Geometry check sheet. Reference: drawing and pictorial views, mm from the part's lowest x, y, z. A direction names the side the tool comes from. Round coordinates to 2 decimals unless told otherwise and drop trailing zeros. Write each loop counter-clockwise with the first axis right and the second up, starting at its lowest first coordinate (ties: lowest second). Pieces come first, ordered by that corner, then holes. Notation, with made-up numbers: M -6.75,17 L 9.25,17 A15 cw 9.25,41 Z; hole C 87.25,-5 d10. An arc over 180 degrees is marked long. Answer in a Markdown table with one row per item. Add a question column.
1. Go/stop test with flat-tipped pins: pin 1 Ø10 at (y, z) = (6, 25) entering from +X; pin 2 Ø6 at (x, z) = (5, 22) entering from -Y; pin 3 Ø12 at (y, z) = (24.5, 28) entering from -X. Record where each tip stops, or that it passes through.
2. Material ranges on probe 1 along Z at (x, y) = (4, 25); probe 2 along Y at (x, z) = (15.5, 33), recorded low to high.
3. Sectioned sample at D-D on z = 36. Record the cut outline in (x, y), plus the area to 3 significant figures.
4. Sectioned sample at C-C on y = 2.5. Record the cut outline in (x, z), plus the area to 3 significant figures.
5. Draft check along Z on the marked faces 3, 4 and 5. Enter one of: pulls with the +Z half, pulls with the -Z half, needs draft (parallel to the pull), parting line crosses it, or undercut.
6. Set-up check for the marked faces 1 and 2: record each of +Z, -Z, +X, -X, +Y, -Y from which the full face is reachable in a straight line by a thin tool's end or side.
7. Sectioned sample at A-A on x = 15. Record the cut outline in (y, z), plus the area to 3 significant figures.
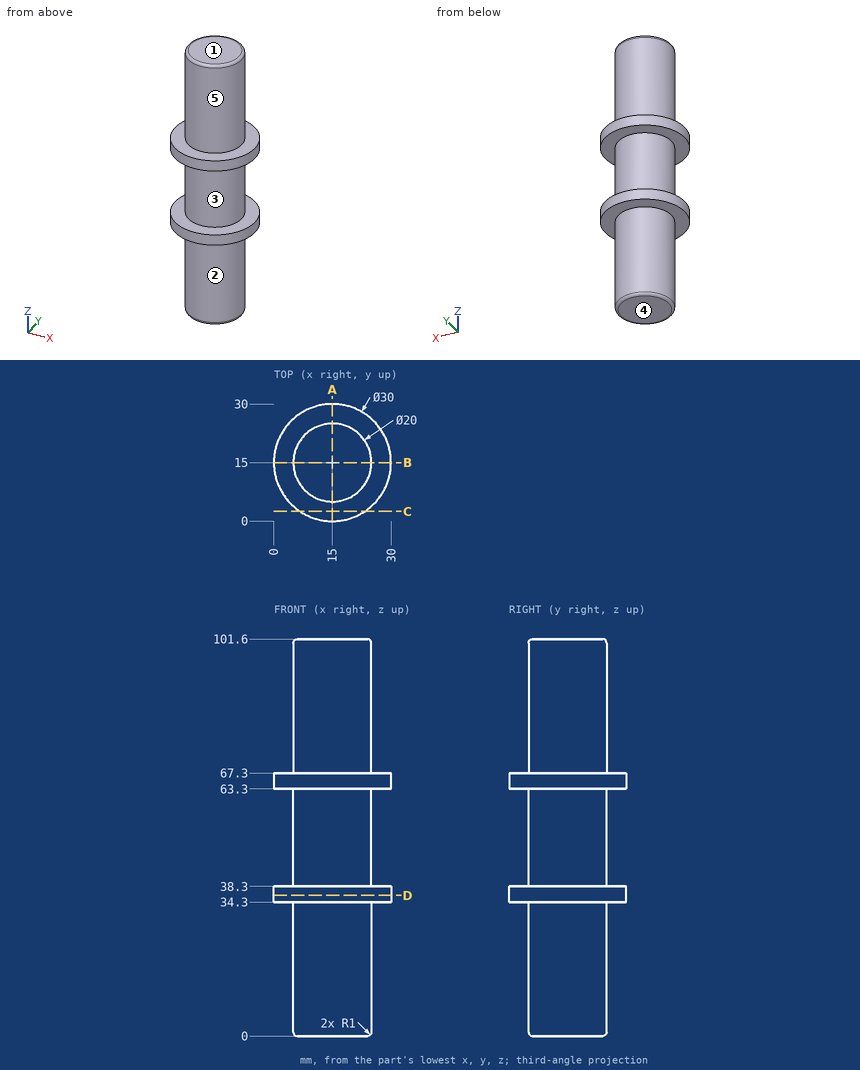
Geometry check:
| question | item | result |
|---|---|---|
| 1 | pin 1 | stops at x = 24.17 |
| 1 | pin 2 | stops at y = 7.86 |
| 1 | pin 3 | stops at x = 5.63 |
| 2 | probe 1 | z = 34.3 to 38.3, 63.3 to 67.3 |
| 2 | probe 2 | y = 5.01 to 24.99 |
| 3 | outline | C 15,15 d30 |
| 3 | area | 707 mm2 |
| 4 | outline | M 6.71,34.3 L 23.29,34.3 L 23.29,38.3 L 6.71,38.3 Z; M 6.71,63.3 L 23.29,63.3 L 23.29,67.3 L 6.71,67.3 Z |
| 4 | area | 133 mm2 |
| 5 | face 3 | undercut |
| 5 | face 4 | pulls with the -Z half |
| 5 | face 5 | needs draft |
| 6 | face 1 | +Z, +X, -X, +Y, -Y |
| 6 | face 2 | -Z |
| 7 | outline | M 0,34.3 L 5,34.3 L 5,1 A1 ccw 6,0 L 24,0 A1 ccw 25,1 L 25,34.3 L 30,34.3 L 30,38.3 L 25,38.3 L 25,63.3 L 30,63.3 L 30,67.3 L 25,67.3 L 25,100.6 A1 ccw 24,101.6 L 6,101.6 A1 ccw 5,100.6 L 5,67.3 L 0,67.3 L 0,63.3 L 5,63.3 L 5,38.3 L 0,38.3 Z |
| 7 | area | 2,110 mm2 |
